Can you work these out from the model? Positions are in its coordinate system, mm. Give positions to 0.01 mm unless a question says otherwise; leave off trailing zeros. Order: outer loops, then holes, each group sorted by start corner. A loop starts at its lowest first (then second) coordinate and runs counter-clockwise, first axis right, second up. Notation, with made-up numbers: M -11,13 L 0,13 A22 ccw 0,22 Z; hole C 54,56.25 d4. An arc over 180 degrees is marked long. Answer as a JSON object with one key per item and string values.
```python
from build123d import *

# Parameters (mm, degrees)
SKETCH1_W           = 200
SKETCH1_H           = 120
SKETCH1_R           = 3.25
SKETCH1_R_2         = 47.625
SKETCH1_R_3         = 2.945643703
BOSS_EXTRUDE1_DEPTH = 3.1
SKETCH2_W           = 3.1
SKETCH2_H           = 60
BOSS_EXTRUDE2_DEPTH = 3.1
SKETCH3_W           = 100
SKETCH3_H           = 3.1
CUT_EXTRUDE1_DEPTH  = 4.1
BOSS_EXTRUDE3_DEPTH = 3.1


with BuildPart() as part:
    # Sketch1 → Boss-Extrude1 (new body)
    with BuildSketch(Plane.XY):
        with Locations((9.675, 0)):
            Rectangle(SKETCH1_W, SKETCH1_H)
        with Locations((-39.522196789, 36.759986207)):
            Circle(SKETCH1_R, mode=Mode.SUBTRACT)
        with Locations((36.759986207, 39.522196789)):
            Circle(SKETCH1_R, mode=Mode.SUBTRACT)
        with Locations((39.522196789, -36.759986207)):
            Circle(SKETCH1_R, mode=Mode.SUBTRACT)
        with Locations((-36.759986207, -39.522196789)):
            Circle(SKETCH1_R, mode=Mode.SUBTRACT)
        Circle(SKETCH1_R_2, mode=Mode.SUBTRACT)
        with Locations((-70.325, 0)):
            Circle(SKETCH1_R_3, mode=Mode.SUBTRACT)
        with Locations((89.675, 0)):
            Circle(SKETCH1_R_3, mode=Mode.SUBTRACT)
    extrude(amount=BOSS_EXTRUDE1_DEPTH)

    # Sketch2 → Boss-Extrude2 (add, through all)
    with BuildSketch(Plane.XY.offset(3.1)):
        with Locations((-91.875, 30)):
            Rectangle(SKETCH2_W, SKETCH2_H)
        with Locations((111.225, 30)):
            Rectangle(SKETCH2_W, SKETCH2_H)
    extrude(amount=-BOSS_EXTRUDE2_DEPTH)

    # Sketch3 → Cut-Extrude1 (cut, through all)
    with BuildSketch(Plane.XY.offset(3.1)):
        with Locations((9.675, -58.45)):
            Rectangle(SKETCH3_W, SKETCH3_H)
        with Locations((9.675, 58.45)):
            Rectangle(SKETCH3_W, SKETCH3_H)
    extrude(amount=-CUT_EXTRUDE1_DEPTH, mode=Mode.SUBTRACT)

    # Sketch4 → Boss-Extrude3 (add, through all)
    with BuildSketch(Plane.XY.offset(3.1)):
        Polygon((112.775, 0), (112.775, -59.080724095), (128.775, -59.080724095), (128.775, 0), (131.875, 0), (131.875, -59.080724095), (136.875, -59.080724095), (136.875, 60), (112.775, 60), align=None)
    extrude(amount=-BOSS_EXTRUDE3_DEPTH)


solid = part.part
```
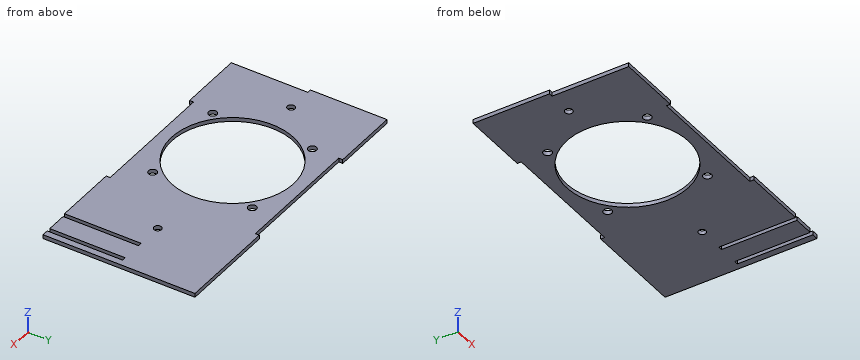
1) I'm going to push flat-ended pins straight in: pin 1 Ø1.5 at (x, z) = (-27.5, 2) entering from -Y; pin 2 Ø1.5 at (y, z) = (-58.5, 1.5) entering from -X (3 decimals); pin 3 Ø6 at (x, y) = (39.52, -36.76) entering from +Z. Where does each tip first touch, or does it pass through?
Results found:
{"pin 1": "stops at y = -56.9", "pin 2": "stops at x = -90.325", "pin 3": "passes through"}
2) I want a section at B-B on z = 2.3. Count the separate pieces of the cut face and the enclosed holes in it, and give its area (3 significant figures).
Results found:
{"separate pieces": "1", "enclosed holes": "7", "area": "19,100 mm²"}
3) I want a section at A-A on x = 0. Write out the boundary of the cut face in (y, z) (3 decimals).
Results found:
{"outline": "M -56.9,0 L -47.625,0 L -47.625,3.1 L -56.9,3.1 Z; M 47.625,0 L 56.9,0 L 56.9,3.1 L 47.625,3.1 Z"}
4) I want a section at C-C on y = -20. Write out the boundary of the cut face in (x, z) (3 decimals), and give its area (3 significant figures).
Results found:
{"outline": "M -90.325,0 L -43.222,0 L -43.222,3.1 L -90.325,3.1 Z; M 43.222,0 L 109.675,0 L 109.675,3.1 L 43.222,3.1 Z; M 112.775,0 L 128.775,0 L 128.775,3.1 L 112.775,3.1 Z; M 131.875,0 L 136.875,0 L 136.875,3.1 L 131.875,3.1 Z", "area": "417 mm²"}
5) I want a section at D-D on x = 57. Write out the boundary of the cut face in (y, z).
Results found:
{"outline": "M -56.9,0 L 56.9,0 L 56.9,3.1 L -56.9,3.1 Z"}
6) I need wall thicknesses on L1, parallel to X at y = -51, z = 1 (3 decimals); L2, parallel to Y at x = 0, z = 1.2 (3 decimals); L3, parallel to Y at x = 42.5, z = 0.65. Which ranges of each line are inside material? Lowest first, please.
Results found:
{"L1": "x = -90.325 to 109.675, 112.775 to 128.775, 131.875 to 136.875", "L2": "y = -56.9 to -47.625, 47.625 to 56.9", "L3": "y = -56.9 to -38.06, -35.46 to -21.49, 21.49 to 56.9"}
